Check sheet for the modelled part. Datum: model origin and axes. Units: mm. A direction names the side the tool comes from. Round coordinates to 2 decimals unless told otherwise and drop trailing zeros. Loops run counter-clockwise (first coordinate to the right, second up) from the corner with the lowest first, then second, coordinate; pieces in that order, holes last. Notation, with made-up numbers: (-9.75, 50.25) - (21.25, 50.25) arc R16 cw to (21.25, 74.25) - close; hole circle Ø10 at (-14, 49). An arc over 180 degrees is marked (long way). Put each result on its own line as item: value. Start each with the question number.
Item 1: Material ranges on line 1 along Z through (x, y) = (27, 68); line 2 along Y through (x, z) = (10, -39.5), recorded low to high.
Item 2: Tool access check on faces 1 (the flat face through (-85.68, 174.67, 1.24)), 2 (the flat face through (88.9, 88, 1)), 3 (the flat face through (-1, 88, -38.1)), 4 (the flat face through (0.62, 174.58, -41.23)), 5 (the flat face through (0.62, 3.22, -41.23)). Record the directions out of +Z, -Z, +X, -X, +Y, -Y that give a thin tool (end or side, any length) a straight path to the whole face; none if there is none.
Item 3: Section check A-A, the plane z = -19. Record the cut outline in (x, y).
Item 4: Section check B-B, the plane y = 130.5. Record the cut outline in (x, z).
Item 5: Draft check along X on faces 6 (the flat face through (-88.9, 88, 1)), 7 (the flat face through (-41.23, 3.22, -0.62)), 8 (the flat face through (-1.24, 3.13, 85.68)). Enter one of: pulls with the +X half, pulls with the -X half, needs draft (parallel to the pull), parting line crosses it, or undercut.
Item 6: Section check C-C, the plane x = 1.5. Record the cut outline in (y, z).
from build123d import *

# Parameters (mm, degrees)
SKETCH2_W               = 177.8
SKETCH2_H               = 177.8
BOSS_EXTRUDE1_DEPTH     = 177.8
CUT_EXTRUDE1_DEPTH      = 218.759638133
CUT_EXTRUDE1_DEPTH_BACK = 218.759638133
SKETCH3_W               = 76.2
SKETCH3_H               = 76.2
CHAMFER1_SIZE           = 6.35


with BuildPart() as part:
    # Sketch2 → Boss-Extrude1 (new body)
    with BuildSketch(Plane(origin=(0, 0, 0), x_dir=(1, 0, 0), z_dir=(0, 1, 0))):
        Rectangle(SKETCH2_W, SKETCH2_H)
    extrude(amount=BOSS_EXTRUDE1_DEPTH)

    # Sketch3 → Cut-Extrude1 (cut, two sides: drawn at the far end of the back side and taken through both)
    with BuildSketch(Plane(origin=(0, 177.8, 0), x_dir=(1, 0, 0), z_dir=(0, 1, 0)).offset(-CUT_EXTRUDE1_DEPTH_BACK)):
        Rectangle(SKETCH3_W, SKETCH3_H)
    extrude(amount=CUT_EXTRUDE1_DEPTH + CUT_EXTRUDE1_DEPTH_BACK, mode=Mode.SUBTRACT)

    # Chamfer1
    chamfer1_edges = [part.edges().sort_by_distance(p)[0] for p in [
        (-88.9, 177.8, 0),
        (0, 177.8, 88.9),
        (38.1, 177.8, 0),
        (38.1, 0, 0),
        (0, 177.8, 38.1),
        (0, 0, 38.1),
        (-38.1, 177.8, 0),
        (-38.1, 0, 0),
        (0, 177.8, -38.1),
        (0, 0, -38.1),
        (88.9, 177.8, 0),
        (0, 0, 88.9),
        (-88.9, 0, 0),
        (0, 0, -88.9),
        (88.9, 0, 0),
        (0, 177.8, -88.9),
    ]]
    chamfer(chamfer1_edges, length=CHAMFER1_SIZE)


solid = part.part
Check result:
1. line 1: -88.9 to -38.1, 38.1 to 88.9
1. line 2: 4.95 to 172.85
2. face 1: +Z, -Z, -X, +Y
2. face 2: +Z, -Z, +X, +Y, -Y
2. face 3: +Y, -Y
2. face 4: +Y
2. face 5: -Y
3. outline: (-88.9, 6.35) - (-82.55, 0) - (-44.45, 0) - (-38.1, 6.35) - (-38.1, 171.45) - (-44.45, 177.8) - (-82.55, 177.8) - (-88.9, 171.45) - close; (38.1, 6.35) - (44.45, 0) - (82.55, 0) - (88.9, 6.35) - (88.9, 171.45) - (82.55, 177.8) - (44.45, 177.8) - (38.1, 171.45) - close
4. outline: (-88.9, -88.9) - (88.9, -88.9) - (88.9, 88.9) - (-88.9, 88.9) - close; hole (-38.1, -38.1) - (38.1, -38.1) - (38.1, 38.1) - (-38.1, 38.1) - close
5. face 6: pulls with the -X half
5. face 7: undercut
5. face 8: needs draft
6. outline: (0, -82.55) - (6.35, -88.9) - (171.45, -88.9) - (177.8, -82.55) - (177.8, -44.45) - (171.45, -38.1) - (6.35, -38.1) - (0, -44.45) - close; (0, 44.45) - (6.35, 38.1) - (171.45, 38.1) - (177.8, 44.45) - (177.8, 82.55) - (171.45, 88.9) - (6.35, 88.9) - (0, 82.55) - close
